Design review of the part built by this model. Coordinates are the model's own, in mm. A direction names the side the tool comes from. Give positions to 0.01 mm unless a question says otherwise; leave off trailing zeros. Order: outer loops, then holes, each group sorted by start corner. A loop starts at its lowest first (then second) coordinate and runs counter-clockwise, first axis right, second up.
Autodesk Inventor part; units mm, degrees
ref_plane "YZ Plane" through (0, 0, 0) normal (1, 0, 0) x (0, 1, 0)
ref_plane "XZ Plane" through (0, 0, 0) normal (0, 1, 0) x (-1, 0, 0)
ref_plane "XY Plane" through (0, 0, 0) normal (0, 0, 1) x (1, 0, 0)
sketch "Sketch1" plane through (0, 0, 0) normal (0, 1, 0) x (-1, 0, 0)
  line L0 (-3, -8) -> (3, -8)
  line L1 (3, -8) -> (3, 8)
  line L2 (3, 8) -> (-3, 8)
  line L3 (-3, 8) -> (-3, -8)
  line L4 (-3, -8) -> (3, 8) construction
  line L5 (3, -8) -> (-3, 8) construction
  point P0 (0, 0)
  dimension "d0" = 16
  dimension "d1" = 6
extrude "Extrusion1" add sketch "Sketch1" along normal blind 2.5
sketch "Sketch2" plane through (0, 2.5, 0) normal (0, 1, 0) x (1, 0, 0)
  line L0 (0, 5) -> (0, 2) construction
  line L1 (-1.25, 5) -> (-1.25, 2)
  line L2 (1.25, 2) -> (1.25, 5)
  arc A0 (1.25, 5) -> (-1.25, 5) centre (0, 5) ccw
  arc A1 (-1.25, 2) -> (1.25, 2) centre (0, 2) ccw
  line L3 (-3, -8) -> (3, -8)
  line L4 (-3, 8) -> (-3, -8)
  line L5 (-3, -8) -> (3, -8)
  line L6 (3, -8) -> (3, 8)
  line L7 (3, 8) -> (-3, 8)
  point P0 (0, 3.5)
  point P1 (0, 3.5)
  dimension "d4" = 2.5
  dimension "d7" = 6
  dimension "d8" = 3
  dimension "d9" = 3
  dimension "d28" = 3
extrude "Extrusion2" cut sketch "Sketch2" against normal through all contours A0 L2 A1 L1
sketch "Sketch3" plane through (3, 0, 8) normal (1, 0, 0) x (0, 0, -1)
  line L0 (16, 0) -> (0, 0)
  line L1 (16, 0) -> (2, 0)
  line L2 (2, 0) -> (2, 1)
  line L3 (2, 1) -> (16, 1)
  line L4 (16, 1) -> (16, 0)
  line L5 (0, 0) -> (0, 2.5)
  line L6 (0, 2.5) -> (16, 2.5)
  point P0 (8, 0)
  point P1 (2, 0)
  dimension "d12" = 2
  dimension "d13" = 1.5
extrude "Extrusion3" cut sketch "Sketch3" against normal through all
sketch "Sketch4" plane through (0, 2.5, 0) normal (0, 1, 0) x (1, 0, 0)
  line L0 (-3, 8) -> (-3, -8)
  line L1 (3, -8) -> (3, 8)
  arc A0 (-3, -6) -> (3, -6) centre (0, -4.75) ccw
  line L2 (-3, -8) -> (3, -8)
  point P0 (0, 0)
  point P1 (-2, 6)
  point P2 (2, 6)
  point P3 (3, 8)
  point P4 (0, -8)
  point P5 (-2.2361, -8)
  dimension "d17" = 2
extrude "Extrusion4" cut sketch "Sketch4" against normal through all
sketch "Sketch5" plane through (0, 2.5, 0) normal (0, 1, 0) x (1, 0, 0)
  line L0 (3, -6) -> (3, 8)
  line L1 (3, 8) -> (-3, 8)
  line L2 (-3, 8) -> (-3, -6)
  arc A0 (1.25, 5) -> (-1.25, 5) centre (0, 5) ccw
  arc A1 (3, 4) -> (0, 7.5) centre (-1.8689, 2.8624) ccw
  arc A2 (0, 7.5) -> (-3, 4) centre (1.8689, 2.8624) ccw
  point P0 (0, 0)
  point P1 (-3, 6.2041)
  point P2 (0, 6.25)
  point P3 (0, 6.25)
  dimension "d23" = 5
  dimension "d24" = 4
  dimension "d25" = 0.5
extrude "Extrusion5" cut sketch "Sketch5" against normal through all
sketch "Sketch6" plane through (-3, 1, 6) normal (0, -1, 0) x (1, 0, 0)
  line L0 (6.1469, -11) -> (-0.0299, -11)
  line L1 (-0.0299, -11) -> (-0.0299, -13.5)
  line L2 (-0.0299, -13.5) -> (6.1469, -13.5)
  line L3 (6.1469, -13.5) -> (6.1469, -11)
  arc A0 (1.75, -11) -> (4.25, -11) centre (3, -11) ccw
  point P0 (3, -6)
  point P1 (3, -13.5)
  point P2 (1.75, -11)
extrude "Extrusion6" cut sketch "Sketch6" against normal blind 0.3 contours L3 L2 L1 L0 A0
sketch "Sketch7" plane through (0, 2.5, 0) normal (0, 1, 0) x (1, 0, 0)
  line L0 (3, -6) -> (3, 4)
  line L1 (-3, 4) -> (-3, -6)
  line L2 (-3, -4.25) -> (3, -4.25)
  arc A0 (-1.25, 2) -> (1.25, 2) centre (0, 2) ccw
  arc A1 (-3, -6) -> (3, -6) centre (0, -4.75) ccw
  point P0 (0, 0)
  point P1 (0, 0.75)
  dimension "d29" = 5
extrude "Extrusion7" cut sketch "Sketch7" against normal through all
fillet "Fillet2" radius 2 2 edges at (3, 1.75, 4.25) (-3, 1.75, 4.25)
sketch "Sketch8" plane through (0, 2.5, 0) normal (0, 1, 0) x (1, 0, 0)
  line L0 (3, -4.25) -> (-3, -4.25)
  line L1 (-3, -4.25) -> (-3, -0.75)
  line L2 (-3, -0.75) -> (3, -0.75)
  line L3 (3, -0.75) -> (3, -4.25)
  arc A0 (-1.25, 2) -> (1.25, 2) centre (0, 2) ccw
  line L4 (3, -2.25) -> (3, 4)
  line L5 (-3, 4) -> (-3, -2.25)
  point P0 (0, 0)
  point P1 (1, -4.25)
  dimension "d33" = 2.75
extrude "Extrusion8" cut sketch "Sketch8" against normal through all
fillet "Fillet3" radius 0.5 2 edges at (3, 1.75, 0.75) (-3, 1.75, 0.75)
properties part number "Carrier Tab 2x2 V1"
1. Take a section at B-B (z = -3). State the section outline as (x, y) points.
Recorded:
outline: (-3, 1) - (-1.25, 1) - (-1.25, 2.5) - (-3, 2.5) - close; (1.25, 1) - (3, 1) - (3, 2.5) - (1.25, 2.5) - close
2. Machinability: for faces 1 (the face through (0, 2, 0.75)), 2 (the face through (-1.25, 2, -4)), 3 (the face through (0, 1.3, -7)), which of the approach directions +Z, -Z, +X, -X, +Y, -Y give a long, thin tool a straight path to every point of the face, cutting with its end or side? Answer none if there is none.
Recorded:
face 1: +Z, +X, -X, +Y, -Y
face 2: +Y, -Y
face 3: -Z, +X, -X, -Y
3. Draft analysis for pull direction X (two halves, no side actions). For faces 4 (the face through (-0.03, 1.76, -0.75)), 5 (the face through (1, 1, -1)), 6 (the face through (-3, 2, -2)), state which applies: pulls with the +X half, pulls with the -X half, needs draft (parallel to the pull), parting line crosses it, or undercut.
Recorded:
face 4: undercut
face 5: needs draft
face 6: pulls with the -X half
4. Take a section at D-D (y = 1.15). State the section outline as (x, z) points, then the cut area to 3 significant figures.
Recorded:
outline: (-3, -4) arc R5 ccw to (-2.65, -5) - (-1.25, -5) - (-1.25, -2) arc R1.25 cw to (1.25, -2) - (1.25, -5) - (2.65, -5) arc R5 ccw to (3, -4) - (3, 0.25) arc R0.5 ccw to (2.5, 0.75) - (-2.5, 0.75) arc R0.5 ccw to (-3, 0.25) - close
area: 24.1 mm2
5. Take a section at A-A (y = 2.35). State the section outline as (x, z) points, then the cut area to 3 significant figures.
Recorded:
outline: (-3, -4) arc R5 ccw to (0, -7.5) arc R5 ccw to (3, -4) - (3, 0.25) arc R0.5 ccw to (2.5, 0.75) - (-2.5, 0.75) arc R0.5 ccw to (-3, 0.25) - close; hole (-1.25, -5) arc R1.25 ccw to (1.25, -5) - (1.25, -2) arc R1.25 ccw to (-1.25, -2) - close
area: 30.0 mm2
6. Take a section at C-C (x = 0.5). State the section outline as (y, z) points, then the cut area to 3 significant figures.
Recorded:
outline: (1, -0.85) - (2.5, -0.85) - (2.5, 0.75) - (1, 0.75) - close; (1.3, -7.27) - (2.5, -7.27) - (2.5, -6.15) - (1.3, -6.15) - close
area: 3.75 mm2
7. For pin 1 (2 mm diameter, centred on x = 0.5, z = -6, fed in from -Y), flat-tipped, find the tip position at first contact; note if it passes through.
Recorded:
pin 1: stops at y = 1.3
8. For line 1 along X through (y, z) = (1.2, -3); line 2 along X through (y, z) = (1.75, -5); line 3 along Z through (x, y) = (-0.5, 1.4), list the stretches that pass through material, from the lowest coordinate up.
Recorded:
line 1: x = -3 to -1.25, 1.25 to 3
line 2: x = -2.65 to -1.25, 1.25 to 2.65
line 3: z = -7.27 to -6.15, -0.85 to 0.75
